from build123d import *

# Parameters (mm, degrees)
BOSS_EXTRUDE1_DEPTH  = 4
CUT_EXTRUDE1_DEPTH   = 3
SKETCH5_W            = 51
SKETCH5_H            = 16
BOSS_EXTRUDE2_DEPTH  = 4
BOSS_EXTRUDE15_DEPTH = 31
SKETCH20_R           = 2.4
CUT_EXTRUDE26_DEPTH  = 1
FILLET8_R            = 4
FILLET12_R           = 8
CUT_EXTRUDE_8_DEPTH  = 29
SKETCH_8_W           = 9
SKETCH_8_H           = 16
CUT_EXTRUDE_10_DEPTH = 8
SKETCH_10_W          = 60
SKETCH_10_H          = 38
EXTRUDE_2_DEPTH      = 8
FILLET_3_R           = 4
FILLET_4_R           = 4
FILLET_5_R           = 4
FILLET_6_R           = 4


with BuildPart() as part:
    # Sketch2 → Boss-Extrude1 (new body)
    with BuildSketch(Plane.XY):
        with BuildLine():
            Line((23.733047461, 11.63962887), (23.733047461, -4.36037113))
            Line((23.733047461, -4.36037113), (-24.266952539, -4.36037113))
            ThreePointArc((-24.266952539, -4.36037113), (-30.597931628, 3.63962887), (-24.266952539, 11.63962887))
            Line((-24.266952539, 11.63962887), (23.733047461, 11.63962887))
        make_face()
    extrude(amount=BOSS_EXTRUDE1_DEPTH)

    # Sketch1 → Cut-Extrude1 (cut)
    with BuildSketch(Plane.XY):
        with BuildLine():
            Line((-6.25004119, 8.63962887), (-20.04279291, 6.23962887))
            ThreePointArc((-20.04279291, 6.23962887), (-22.105421524, 3.63962887), (-20.04279291, 1.03962887))
            Line((-20.04279291, 1.03962887), (-6.25004119, -1.36037113))
            ThreePointArc((-6.25004119, -1.36037113), (-2.105421524, -2.86037113), (2.039198142, -1.36037113))
            Line((2.039198142, -1.36037113), (15.831949862, 1.03962887))
            ThreePointArc((15.831949862, 1.03962887), (17.894578476, 3.63962887), (15.831949862, 6.23962887))
            Line((15.831949862, 6.23962887), (2.039198142, 8.63962887))
            ThreePointArc((2.039198142, 8.63962887), (-2.105421524, 10.13962887), (-6.25004119, 8.63962887))
        make_face()
    extrude(amount=CUT_EXTRUDE1_DEPTH, mode=Mode.SUBTRACT)

    # Sketch5 → Boss-Extrude2 (add)
    with BuildSketch(Plane(origin=(23.733047461, 0, 0), x_dir=(0, 0, -1), z_dir=(1, 0, 0))):
        with Locations((21.5, 3.63962887)):
            Rectangle(SKETCH5_W, SKETCH5_H)
    extrude(amount=BOSS_EXTRUDE2_DEPTH)

    # Sketch6 → Boss-Extrude15 (add)
    with BuildSketch(Plane(origin=(0, 0, -47), x_dir=(-1, 0, 0), z_dir=(0, 0, -1))):
        Polygon((-30.946192459, -15.36037113), (-83.733047461, -15.36037113), (-83.733047461, 22.63962887), (-23.733047461, 22.63962887), (-23.733047461, -15.36037113), align=None)
    extrude(amount=-BOSS_EXTRUDE15_DEPTH)

    # Sketch20 → Cut-Extrude26 (cut)
    with BuildSketch(Plane(origin=(0, 0, 3), x_dir=(-1, 0, 0), z_dir=(0, 0, -1))):
        with Locations((2.105421524, 3.63962887)):
            Circle(SKETCH20_R)
    extrude(amount=-CUT_EXTRUDE26_DEPTH, mode=Mode.SUBTRACT)

    # Fillet8
    fillet8_edges = [part.edges().sort_by_distance(p)[0] for p in [
        (23.733047461, 3.63962887, 0),
    ]]
    fillet(fillet8_edges, radius=FILLET8_R)

    # Fillet12
    fillet12_edges = [part.edges().sort_by_distance(p)[0] for p in [
        (27.733047461, 3.63962887, 4),
    ]]
    fillet(fillet12_edges, radius=FILLET12_R)

    # Sketch 5 → Cut-Extrude 8 (cut)
    with BuildSketch(Plane.XY.offset(-16)):
        Polygon((75.733047461, -7.806095257), (75.733047461, 14.193904743), (33.733047461, 14.193904743), (33.733047461, 3.193904743), (33.733047461, -7.806095257), align=None)
    extrude(amount=-CUT_EXTRUDE_8_DEPTH, mode=Mode.SUBTRACT)

    # Sketch 8 → Cut-Extrude 10 (cut)
    with BuildSketch(Plane(origin=(83.733047461, 0, 0), x_dir=(0, 0, -1), z_dir=(1, 0, 0))):
        with Locations((39.5, 3.238584995)):
            Rectangle(SKETCH_8_W, SKETCH_8_H)
    extrude(amount=-CUT_EXTRUDE_10_DEPTH, mode=Mode.SUBTRACT)

    # Sketch 10 → Extrude 2 (add)
    with BuildSketch(Plane(origin=(0, 0, -47), x_dir=(-1, 0, 0), z_dir=(0, 0, -1))):
        with Locations((-53.733047461, 3.63962887)):
            Rectangle(SKETCH_10_W, SKETCH_10_H)
    extrude(amount=EXTRUDE_2_DEPTH)

    # Fillet 3
    fillet_3_edges = [part.edges().sort_by_distance(p)[0] for p in [
        (53.733047461, 22.63962887, -55),
    ]]
    fillet(fillet_3_edges, radius=FILLET_3_R)

    # Fillet 4
    fillet_4_edges = [part.edges().sort_by_distance(p)[0] for p in [
        (53.733047461, -15.36037113, -55),
    ]]
    fillet(fillet_4_edges, radius=FILLET_4_R)

    # Fillet 5
    fillet_5_edges = [part.edges().sort_by_distance(p)[0] for p in [
        (83.733047461, 3.63962887, -55),
        (83.733047461, -15.36037113, -33.5),
        (83.733047461, 22.63962887, -33.5),
    ]]
    fillet(fillet_5_edges, radius=FILLET_5_R)

    # Fillet 6
    fillet_6_edges = [part.edges().sort_by_distance(p)[0] for p in [
        (23.733047461, 3.63962887, -55),
        (23.733047461, 22.63962887, -33.5),
        (23.733047461, -15.36037113, -33.5),
    ]]
    fillet(fillet_6_edges, radius=FILLET_6_R)


solid = part.part
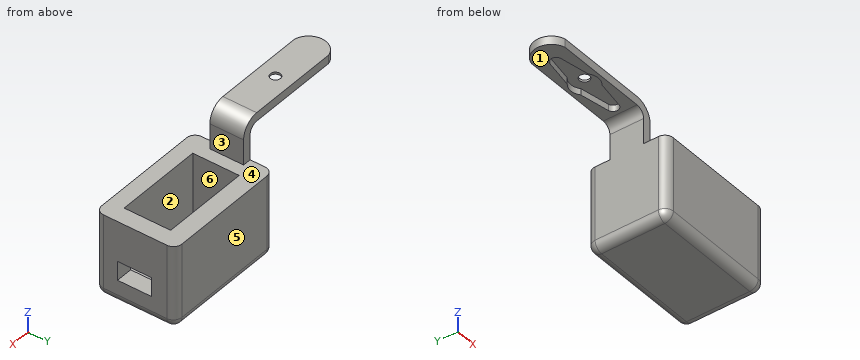
For this review, take the finished solid that the model builds, in its own axes (mm). Face numbers are marked on the shaded views. A direction names the side the tool comes from. Give positions to 0.01 mm unless a question says otherwise; leave off trailing zeros. Order: outer loops, then holes, each group sorted by start corner. A loop starts at its lowest first (then second) coordinate and runs counter-clockwise, first axis right, second up. Notation, with made-up numbers: (-33.5, -8.75) - (-18.5, -8.75) arc R7 ccw to (-18.5, 3.25) - close; hole circle Ø2 at (73.25, 83.25). An arc over 180 degrees is marked (long way). Answer as a JSON object with one key per item and string values. Group by question number.
Item 1: Machinability: for the marked faces 1, 2 and 3, which of the approach directions +Z, -Z, +X, -X, +Y, -Y give a long, thin tool a straight path to every point of the face, cutting with its end or side? Answer none if there is none.
Item 2: Take a section at A-A on z = -19. Give the boundary of the cut face in (x, y).
Item 3: Take a section at C-C on x = 54. Give the boundary of the cut face in (y, z), and give its area (3 significant figures).
Item 4: Clearance check with flat-ended pins moving along their axes: pin 1 Ø6 at (x, y) = (12, 15) entering from +Z; pin 2 Ø6.5 at (x, y) = (78.5, 5.5) entering from +Z; pin 3 Ø8 at (y, z) = (11, -46) entering from -X; pin 4 Ø3 at (y, z) = (-2.5, -41.5) entering from +X. State where each tip first meets the part, or that it passes through.
Item 5: Draft analysis for pull direction Y (two halves, no side actions). For the marked faces 4, 5 and 6, state which applies: pulls with the +Y half, pulls with the -Y half, needs draft (parallel to the pull), parting line crosses it, or undercut.
Item 6: Wall thickness on line 1 along Y through (x, z) = (36.5, -22); line 2 along X through (y, z) = (-3.5, -33); line 3 along Z through (x, y) = (28, 5.5): over which ranges is each line inside the solid? List them lowest first.
Item 7: Take a section at B-B on z = -41.5. Give the boundary of the cut face in (x, y).
Item 8: Take a section at D-D on x = 10.5. Give the boundary of the cut face in (y, z), and give its area (3 significant figures).
Reported:
{
 "1": {"face 1": "-Z, -X, +Y, -Y", "face 2": "+Z", "face 3": "+Z, +X, +Y, -Y"},
 "2": {"outline": "(23.73, -11.36) arc R4 ccw to (27.73, -15.36) - (79.73, -15.36) arc R4 ccw to (83.73, -11.36) - (83.73, 18.64) arc R4 ccw to (79.73, 22.64) - (27.73, 22.64) arc R4 ccw to (23.73, 18.64) - close; hole (33.73, -7.81) - (75.73, -7.81) - (75.73, 14.19) - (33.73, 14.19) - close"},
 "3": {"outline": "(-15.36, -51) arc R4 ccw to (-11.36, -55) - (18.64, -55) arc R4 ccw to (22.64, -51) - (22.64, -16) - (14.19, -16) - (14.19, -45) - (-7.81, -45) - (-7.81, -16) - (-15.36, -16) - close", "area": "837 mm^2"},
 "4": {"pin 1": "through", "pin 2": "z = -16", "pin 3": "x = 23.73", "pin 4": "x = 33.73"},
 "5": {"face 4": "needs draft", "face 5": "pulls with the +Y half", "face 6": "undercut"},
 "6": {"line 1": "-15.36 to -7.81, 14.19 to 22.64", "line 2": "23.73 to 33.73, 75.73 to 83.73", "line 3": "-55 to -16"},
 "7": {"outline": "(23.73, -11.36) arc R4 ccw to (27.73, -15.36) - (79.73, -15.36) arc R4 ccw to (83.73, -11.36) - (83.73, -4.76) - (75.73, -4.76) - (75.73, -7.81) - (33.73, -7.81) - (33.73, 14.19) - (75.73, 14.19) - (75.73, 11.24) - (83.73, 11.24) - (83.73, 18.64) arc R4 ccw to (79.73, 22.64) - (27.73, 22.64) arc R4 ccw to (23.73, 18.64) - close"},
 "8": {"outline": "(-4.36, 0) - (0.11, 0) - (0.11, 3) - (7.17, 3) - (7.17, 0) - (11.64, 0) - (11.64, 4) - (-4.36, 4) - close", "area": "42.8 mm^2"}
}
